Source: three-view drawing plus pictorial views. Frame: mm from the lowest corner of the part. A direction names the side the tool comes from. Give positions to 0.01 mm unless a question says otherwise; leave off trailing zeros. Loops run counter-clockwise (first coordinate to the right, second up) from the corner with the lowest first, then second, coordinate; pieces in that order, holes last. Notation, with made-up numbers: (-20, 75) - (-1, 75) arc R20 cw to (-1, 109) - close; hole circle Ø1 at (-4, 85). An arc over 180 degrees is marked (long way). Put each result on its own line as item: value.
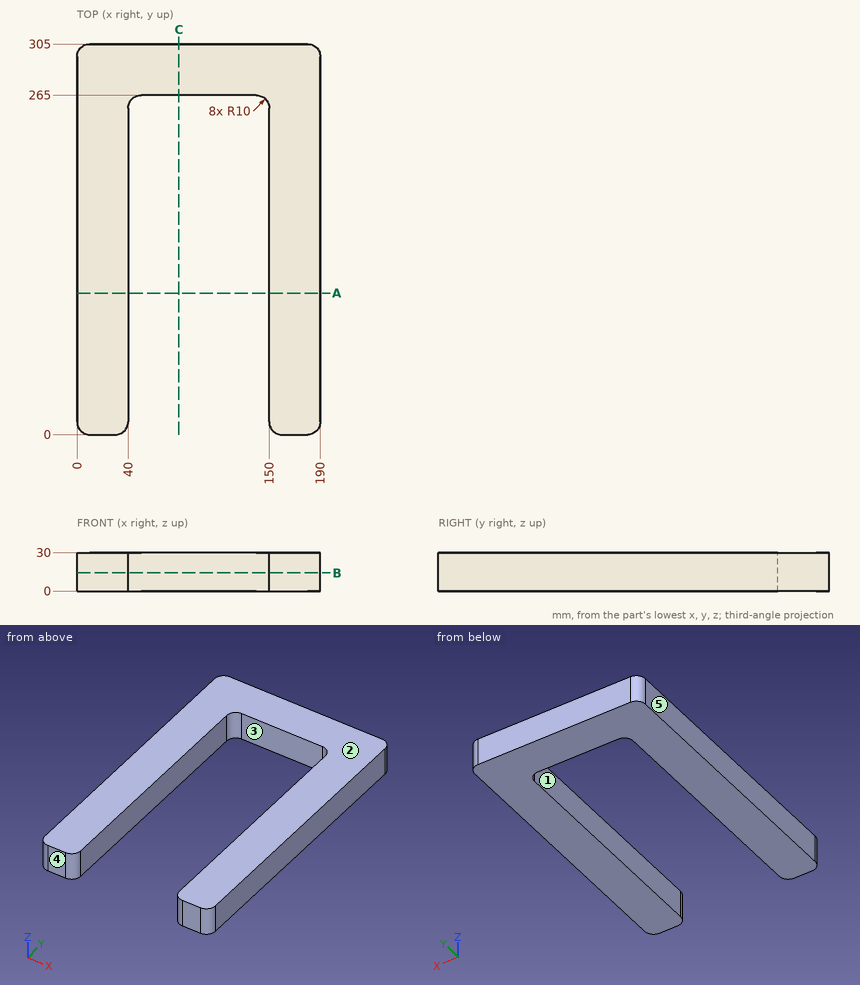
1) Pin query (flat end, axial travel): P1, Ø15, axis at x = 75, z = 19.5, coming from the -Y side; P2, Ø12, axis at y = 65.5, z = 15.5, coming from the -X side; P3, Ø10, axis at x = 43, z = 24, coming from the -Y side; P4, Ø4, axis at x = 50.5, z = 27, coming from the -Y side. Return the tip coordinate at first contact, or that it passes through.
Check result:
P1: y = 265
P2: x = 0
P3: y = 4
P4: y = 264.89
2) Section query B-B, the plane z = 14.25. Output: boundary loops of the cut face in (x, y).
Check result:
outline: (0, 10) arc R10 ccw to (10, 0) - (30, 0) arc R10 ccw to (40, 10) - (40, 255) arc R10 cw to (50, 265) - (140, 265) arc R10 cw to (150, 255) - (150, 10) arc R10 ccw to (160, 0) - (180, 0) arc R10 ccw to (190, 10) - (190, 295) arc R10 ccw to (180, 305) - (10, 305) arc R10 ccw to (0, 295) - close
3) Material intervals for line 1 along X through (y, z) = (54, 15.5); line 2 along Y through (x, z) = (102, 8.75); line 3 along Y through (x, z) = (147, 25.5), sorted ascending. Write a range as [from, to].
Check result:
line 1: [0, 40], [150, 190]
line 2: [265, 305]
line 3: [262.14, 305]
4) Section query C-C, the plane x = 79.5. Output: boundary loops of the cut face in (y, z).
Check result:
outline: (265, 0) - (305, 0) - (305, 30) - (265, 30) - close
5) Access query for the marked faces 1 and 2. Directions: +Z, -Z, +X, -X, +Y, -Y. A direction counts if a zero-diameter tool reaches every point of the face in a straight line with its end or side. Return the directions, or none.
Check result:
face 1: +Z, -Z, -Y
face 2: +Z, +X, -X, +Y, -Y
6) Mould query, pull axis X, two halves, no side actions, for the marked faces 3, 4 and 5. Classes: pulls with the +X half, pulls with the -X half, needs draft (parallel to the pull), parting line crosses it, or undercut.
Check result:
face 3: undercut
face 4: needs draft
face 5: pulls with the -X half
7) Section query A-A, the plane y = 110.5. Output: boundary loops of the cut face in (x, z), plus the area to 3 significant figures.
Check result:
outline: (0, 0) - (40, 0) - (40, 30) - (0, 30) - close; (150, 0) - (190, 0) - (190, 30) - (150, 30) - close
area: 2,400 mm²
